Check sheet for the modelled part. Datum: model origin and axes. Units: mm. Face numbers are marked on the shaded views. A direction names the side the tool comes from. Give positions to 0.01 mm unless a question says otherwise; leave off trailing zeros. Order: outer loops, then holes, each group sorted by start corner. A loop starts at its lowest first (then second) coordinate and runs counter-clockwise, first axis right, second up.
from build123d import *

# Parameters (mm, degrees)
F1_DEPTH = 10
F2_DEPTH = 17
F3_W     = 100
F3_H     = 35
F4_DEPTH = 3
F5_SIZE2 = 10
F5_SIZE  = 100
F6_SIZE2 = 99.99999
F6_SIZE  = 7.49999
F7_R     = 10


# Not quite as in the source:
# - a fillet or chamfer is up to 0.001 mm smaller than in the source, because OpenCascade refuses the exact size


with BuildPart() as f1:
    # F0 (on Top) → F1 (new body)
    with BuildSketch(Plane.XY):
        Polygon((-58.5, -8.5), (-58.5, -2.5), (-58.5, 0), (-58.5, 2.5), (-58.5, 8.5), (-63.5, 0), align=None)
        Polygon((-58.5, -2.5), (-55, -2.5), (-55, 2.5), (-58.5, 2.5), (-58.5, 0), align=None)
    extrude(amount=F1_DEPTH)

    # F0 (on Top) → F2 (join)
    with BuildSketch(Plane.XY):
        Polygon((-55, -17.5), (55, -17.5), (55, 17.5), (-55, 17.5), (-55, 2.5), (-55, -2.5), align=None)
    extrude(amount=F2_DEPTH)

    # F3 (on face) → F4 (join)
    with BuildSketch(Plane.XY.offset(17)):
        with Locations((5, 0)):
            Rectangle(F3_W, F3_H)
    extrude(amount=F4_DEPTH)

    # F5
    f5_edges = [f1.edges().sort_by_distance(p)[0] for p in [
        (55, 0, 0),
    ]]
    f5_side = f1.faces().sort_by_distance((-0.907982, 0, 0))[0]
    chamfer(f5_edges, length=F5_SIZE, length2=F5_SIZE2, reference=f5_side)

    # F6 (size 7.5 and 100 in the source; OpenCascade refuses exactly that, so slightly less here)
    f6_edges = [f1.edges().sort_by_distance(p)[0] for p in [
        (55, -17.5, 15),
        (55, 17.5, 15),
    ]]
    f6_side = f1.faces().sort_by_distance((55, 0, 15))[0]
    chamfer(f6_edges, length=F6_SIZE, length2=F6_SIZE2, reference=f6_side)

    # F7
    f7_edges = [f1.edges().sort_by_distance(p)[0] for p in [
        (55, -10.00001, 15),
        (55, 10.00001, 15),
    ]]
    fillet(f7_edges, radius=F7_R)


solid = f1.part
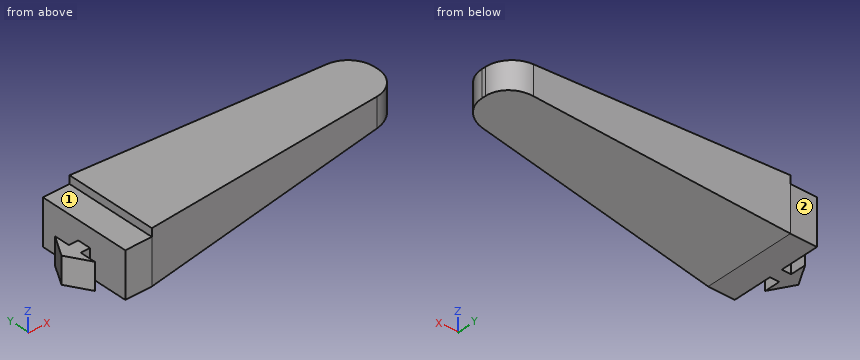
1) Section check A-A, the plane y = 4.5. Record the cut outline in (x, z), then the cut area to 3 significant figures.
Recorded:
outline: (-60.85, 0) - (-58.5, 0) - (-58.5, 10) - (-60.85, 10) - close; (-55, 0) - (-45, 0) - (54.26, 9.93) - (54.26, 20) - (-45, 20) - (-45, 17) - (-55, 17) - close
area: 1,690 mm2
2) Depth check by flat-ended pin: pin 1 Ø5 at (y, z) = (-0.5, 9.5) entering from -X; pin 2 Ø4 at (x, y) = (-57.5, -3) entering from +Z; pin 3 Ø1.5 at (x, y) = (22, -12.5) entering from -Z (3 decimals); pin 4 Ø5 at (x, y) = (-1, -5) entering from -Z. Enter the tip coordinate at first touch or a pass-through.
Recorded:
pin 1: stops at x = -63.5
pin 2: stops at z = 10
pin 3: stops at z = 6.625
pin 4: stops at z = 4.15
3) Material ranges on L1, parallel to Z at x = -46, y = 10.5; L2, parallel to Y at x = -42, z = 16.5 (3 decimals); L3, parallel to X at y = -1, z = 14, recorded low to high.
Recorded:
L1: z = 0 to 17
L2: y = -17.275 to 17.275
L3: x = -55 to 55
4) Section check C-C, the plane x = -5. Record the cut outline in (y, z), then the cut area to 3 significant figures.
Recorded:
outline: (-14.5, 4) - (14.5, 4) - (14.5, 20) - (-14.5, 20) - close
area: 464 mm2
5) Section check B-B, the plane z = 2. Record the cut outline in (x, y), then the cut area to 3 significant figures.
Recorded:
outline: (-63.5, 0) - (-58.5, -8.5) - (-58.5, -2.5) - (-55, -2.5) - (-55, -17.5) - (-45, -17.5) - (-25, -16) - (-25, 16) - (-45, 17.5) - (-55, 17.5) - (-55, 2.5) - (-58.5, 2.5) - (-58.5, 8.5) - close
area: 1,080 mm2
6) Set-up check for the marked faces 1 and 2: record each of +Z, -Z, +X, -X, +Y, -Y from which the full face is reachable in a straight line by a thin tool's end or side.
Recorded:
face 1: +Z, -X, +Y, -Y
face 2: +Z, -Z, +X, -X, +Y
7) Section check D-D, the plane y = -15. Record the cut outline in (x, z).
Recorded:
outline: (-55, 0) - (-45, 0) - (-11.67, 3.33) - (-11.67, 20) - (-45, 20) - (-45, 17) - (-55, 17) - close
